Could you check a few things on this drawing? It's one solid part, dimensions in mm from its lowest x, y, z. Give positions to 0.01 mm unless a question says otherwise; leave off trailing zeros. Loops run counter-clockwise (first coordinate to the right, second up) from the corner with the lowest first, then second, coordinate; pieces in that order, holes last.
Q1. I need wall thicknesses on probe 1 along X at (y, z) = (3, 1.65); probe 2 along X at (y, z) = (22.5, 0.35) (1 decimal); probe 3 along Y at (x, z) = (36, 0.45) (1 decimal). Which ranges of each line are inside material? Lowest first, please.
Q2. Suppose I cut it at B-B (x = 27). List the corners of the cut face in (y, z) for me (1 decimal).
Q3. I'm going to push flat-ended pins straight in: P1, Ø1.6, axis at y = 24, z = 1, coming from the +X side (1 decimal); P2, Ø1.6, axis at x = 86.5, z = 1, coming from the -Y side (1 decimal); P3, Ø1, axis at x = 85.5, z = 2, coming from the +Y side (1 decimal). Where does each tip first touch, or does it pass through?
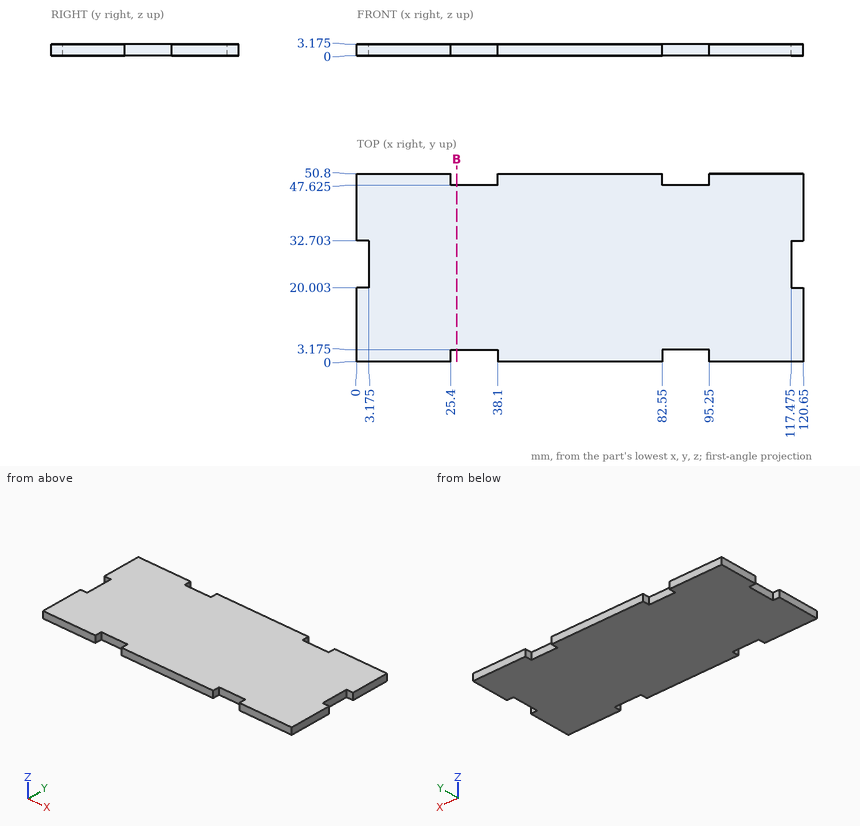
Solutions:
1. probe 1: x = 0 to 25.4, 38.1 to 82.55, 95.25 to 120.65
1. probe 2: x = 3.2 to 117.5
1. probe 3: y = 3.2 to 47.6
2. outline: (3.2, 0) - (47.6, 0) - (47.6, 3.2) - (3.2, 3.2) - close
3. P1: stops at x = 117.5
3. P2: stops at y = 3.2
3. P3: stops at y = 47.6
